from build123d import *

# Parameters (mm, degrees)
BOSS_EXTRUDE1_DEPTH = 38.1
SKETCH2_R           = 4
CUT_EXTRUDE1_DEPTH  = 40.315338398
SKETCH3_W           = 2.032
SKETCH3_H           = 1.1938
CUT_EXTRUDE2_DEPTH  = 40.315338398


with BuildPart() as part:
    # Sketch1 → Boss-Extrude1 (new body)
    with BuildSketch(Plane(origin=(0, 0, 0), x_dir=(0, 0, -1), z_dir=(1, 0, 0))):
        Polygon((7.332348419, 0), (3.666174209, 6.35), (-3.666174209, 6.35), (-7.332348419, 0), (-3.666174209, -6.35), (3.666174209, -6.35), align=None)
    extrude(amount=BOSS_EXTRUDE1_DEPTH)

    # Sketch2 → Cut-Extrude1 (cut, through all)
    with BuildSketch(Plane(origin=(38.1, 0, 0), x_dir=(0, 0, -1), z_dir=(1, 0, 0))):
        Circle(SKETCH2_R)
    extrude(amount=-CUT_EXTRUDE1_DEPTH, mode=Mode.SUBTRACT)

    # Sketch3 → Cut-Extrude2 (cut, through all)
    with BuildSketch(Plane.ZY):
        with Locations((0, 4)):
            Rectangle(SKETCH3_W, SKETCH3_H)
    extrude(amount=-CUT_EXTRUDE2_DEPTH, mode=Mode.SUBTRACT)


solid = part.part
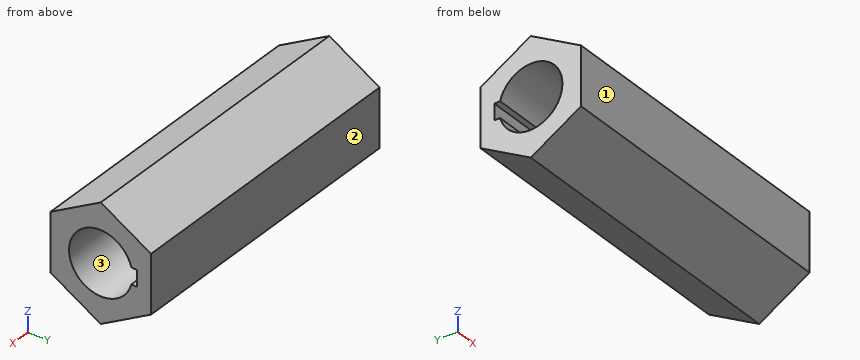
Input: part model. Units: mm. Frame: model coordinates. Face numbers are marked on the shaded views. Coordinates: 2 decimals unless noted, no trailing zeros. Loops run counter-clockwise (first coordinate to the right, second up) from the corner with the lowest first, then second, coordinate; pieces in that order, holes last. Notation, with made-up numbers: (-30.5, 36.25) - (-13.5, 36.25) arc R27 cw to (-13.5, 56.25) - close; hole circle Ø10 at (-33, 75). An arc over 180 degrees is marked (long way). Answer in a Markdown table with one row per item. Add a question column.
Item 1: Section query A-A on z = 0. Return the cut outline in (x, y), then the cut area to 3 significant figures.
Item 2: Line query: line 1 along Y through (x, z) = (27.5, 0); line 2 along Z through (x, y) = (29, 0); line 3 along Z through (x, y) = (27, 3.5). Output: solid intervals per line, ascending. Write a range as [from, to].
Item 3: Section query D-D on z = -5.25. Return the cut outline in (x, y), then the cut area to 3 significant figures.
Item 4: Section query B-B on y = -3. Return the cut outline in (x, z), then the cut area to 3 significant figures.
Item 5: Contact query for flat-ended pins moving along their axis: P1, Ø2, axis at y = -2, z = -3, coming from the -X side; P2, Ø6, axis at x = 26.5, y = 4, coming from the +Z side (3 decimals); P3, Ø2, axis at x = 28.5, z = 5.5, coming from the +Y side; P4, Ø6, axis at x = 18.5, y = -2, coming from the -Z side. Output: stop coordinate, or through.
Item 6: Mould query, pull axis Y, two halves, no side actions, for the marked faces 1, 2 and 3. Classes: released by +Y, released by -Y, zero draft, split by the parting line, or undercut.
Item 7: Section query C-C on x = 10.5. Return the cut outline in (y, z).
Recorded:
| question | item | result |
|---|---|---|
| 1 | outline | (0, -6.35) - (38.1, -6.35) - (38.1, -4) - (0, -4) - close; (0, 4.6) - (38.1, 4.6) - (38.1, 6.35) - (0, 6.35) - close |
| 1 | area | 156 mm^2 |
| 2 | line 1 | [-6.35, -4], [4.6, 6.35] |
| 2 | line 2 | [-7.33, -4], [4, 7.33] |
| 2 | line 3 | [-5.31, -1.94], [1.94, 5.31] |
| 3 | outline | (0, -3.61) - (38.1, -3.61) - (38.1, 3.61) - (0, 3.61) - close |
| 3 | area | 275 mm^2 |
| 4 | outline | (0, -5.6) - (38.1, -5.6) - (38.1, -2.65) - (0, -2.65) - close; (0, 2.65) - (38.1, 2.65) - (38.1, 5.6) - (0, 5.6) - close |
| 4 | area | 225 mm^2 |
| 5 | P1 | x = 0 |
| 5 | P2 | z = 6.755 |
| 5 | P3 | y = 4.91 |
| 5 | P4 | z = -7.33 |
| 6 | face 1 | released by -Y |
| 6 | face 2 | released by +Y |
| 6 | face 3 | undercut |
| 7 | outline | (-6.35, -3.67) - (0, -7.33) - (6.35, -3.67) - (6.35, 3.67) - (0, 7.33) - (-6.35, 3.67) - close; hole (3.87, -1.02) - (4.6, -1.02) - (4.6, 1.02) - (3.87, 1.02) arc R4 ccw (long way) to start |
